from build123d import *

# Parameters (mm, degrees)
F1_DEPTH = 660.4
F2_R     = 6.35
F3_DEPTH = 50.801


with BuildPart() as f1:
    # F0 (on Front) → F1 (new body, symmetric)
    with BuildSketch(Plane.XZ):
        with BuildLine():
            Line((-19.05, -25.4), (19.05, -25.4))
            ThreePointArc((19.05, -25.4), (23.540128, -23.540128), (25.4, -19.05))
            Line((25.4, -19.05), (25.4, 19.05))
            ThreePointArc((25.4, 19.05), (23.540128, 23.540128), (19.05, 25.4))
            Line((19.05, 25.4), (-19.05, 25.4))
            ThreePointArc((-19.05, 25.4), (-23.540128, 23.540128), (-25.4, 19.05))
            Line((-25.4, 19.05), (-25.4, -19.05))
            ThreePointArc((-25.4, -19.05), (-23.540128, -23.540128), (-19.05, -25.4))
        make_face()
        with BuildLine():
            Line((-19.05, 22.225), (19.05, 22.225))
            ThreePointArc((19.05, 22.225), (21.295064, 21.295064), (22.225, 19.05))
            Line((22.225, 19.05), (22.225, -19.05))
            ThreePointArc((22.225, -19.05), (21.295064, -21.295064), (19.05, -22.225))
            Line((19.05, -22.225), (-19.05, -22.225))
            ThreePointArc((-19.05, -22.225), (-21.295064, -21.295064), (-22.225, -19.05))
            Line((-22.225, -19.05), (-22.225, 19.05))
            ThreePointArc((-22.225, 19.05), (-21.295064, 21.295064), (-19.05, 22.225))
        make_face(mode=Mode.SUBTRACT)
    extrude(amount=F1_DEPTH, both=True)

    # F2 (on face) → F3 (cut, through all)
    with BuildSketch(Plane.XY.offset(25.4)):
        Circle(F2_R)
        with Locations((0, -609.6)):
            Circle(F2_R)
        with Locations((0, 609.6)):
            Circle(F2_R)
    extrude(amount=-F3_DEPTH, mode=Mode.SUBTRACT)


solid = f1.part
For this review, take the finished solid that the model builds, in its own axes (mm). A direction names the side the tool comes from. Give positions to 0.01 mm unless a question says otherwise; leave off trailing zeros. Order: outer loops, then holes, each group sorted by start corner. A loop starts at its lowest first (then second) coordinate and runs counter-clockwise, first axis right, second up. Notation, with made-up numbers: M -22.5,70 L 20.5,70 A20 ccw 20.5,74 Z; hole C 12,46.25 d11. An arc over 180 degrees is marked long. Answer in a Markdown table with one row per item. Add a question column.
(1) Mouldability with a two-part tool opening along Z and no side actions: class faces 3 (the face through (22.225, -9, 0)), 4 (the face through (-0.1, -660.4, -22.5)), 5 (the face through (0, -9, 25.4)) as +Z half, -Z half, draft (parallel to the pull), parting line (faces both ways), or undercut.
(2) Wall thickness on probe 1 along Y at (x, z) = (0, 24); probe 2 along Z at (x, y) = (-18, -31) (3 decimals): over which ranges is each line inside the solid? List them lowest first. Write a range as [from, to].
(3) Consider section A-A on z = 10.5. State the section outline as (x, y) points (3 decimals), and give its area (3 significant figures).
(4) Consider section B-B on y = -398.5. State the section outline as (x, z) points (3 decimals), and give its area (3 significant figures).
(5) For faces 1 (the face through (0, -9, 22.225)), 2 (the face through (0, -9, -25.4)), list the 3-axis set-ups (+Z, -Z, +X, -X, +Y, -Y) from which the entire face can be reached by the end or side of a thin tool; tool diameter is ignored.
Evaluation:
| question | item | result |
|---|---|---|
| 1 | face 3 | undercut |
| 1 | face 4 | draft |
| 1 | face 5 | +Z half |
| 2 | probe 1 | y = [-660.4, -615.95], [-603.25, -6.35], [6.35, 603.25], [615.95, 660.4] |
| 2 | probe 2 | z = [-25.4, -22.225], [22.225, 25.4] |
| 3 | outline | M -25.4,-660.4 L -22.225,-660.4 L -22.225,660.4 L -25.4,660.4 Z; M 22.225,-660.4 L 25.4,-660.4 L 25.4,660.4 L 22.225,660.4 Z |
| 3 | area | 8,390 mm^2 |
| 4 | outline | M -25.4,-19.05 A6.35 ccw -19.05,-25.4 L 19.05,-25.4 A6.35 ccw 25.4,-19.05 L 25.4,19.05 A6.35 ccw 19.05,25.4 L -19.05,25.4 A6.35 ccw -25.4,19.05 Z; hole M -22.225,-19.05 A3.175 ccw -19.05,-22.225 L 19.05,-22.225 A3.175 ccw 22.225,-19.05 L 22.225,19.05 A3.175 ccw 19.05,22.225 L -19.05,22.225 A3.175 ccw -22.225,19.05 Z |
| 4 | area | 579 mm^2 |
| 5 | face 1 | +Y, -Y |
| 5 | face 2 | -Z, +X, -X, +Y, -Y |
